Model file for the job. Use its own axes, mm. Face numbers are marked on the shaded views. A direction names the side the tool comes from. Coordinates: 2 decimals unless noted, no trailing zeros. Write each loop counter-clockwise with the first axis right and the second up, starting at its lowest first coordinate (ties: lowest second). Pieces come first, ordered by that corner, then holes.
Q1. Pin check, flat tips, straight feed: P1, Ø4, axis at x = 37, z = -152.5, coming from the -Y side; P2, Ø1, axis at x = -15.5, y = 946, coming from the +Z side. Stop position of each tip, or through.
Q2. Band-saw the part on C-C, the plane x = 33. Write the cut outline in (y, z), plus the area to 3 significant figures.
Q3. Band-saw the part on B-B, the plane y = 1525. Write the cut outline in (x, z), plus the area to 3 significant figures.
Q4. Pull direction X, two halves, no side cores. Call the marked faces 1, 2 and 3: released by +X, released by -X, zero draft, split by the parting line, or undercut.
Q5. Drill centre lines: probe 1 along Y at (x, z) = (62, -112); probe 2 along X at (y, z) = (1181, -19.5); probe 3 along Z at (x, y) = (-39.5, 1463). Where is each one in solid material? Low to high.
Q6. Band-saw the part on A-A, the plane z = -28.5. Write the cut outline in (x, y).
Q7. Which spindle directions (+Z, -Z, +X, -X, +Y, -Y) get a long thin tool onto all of the face, cutting with end or side? Do the marked faces 4 and 5. Say none if no direction does.
Autodesk Inventor part; units mm, degrees
ref_plane "YZ Plane" through (0, 0, 0) normal (1, 0, 0) x (0, 1, 0)
ref_plane "XZ Plane" through (0, 0, 0) normal (0, 1, 0) x (-1, 0, 0)
ref_plane "XY Plane" through (0, 0, 0) normal (0, 0, 1) x (1, 0, 0)
sketch "Schizzo1" plane through (0, 0, 0) normal (0, 0, 1) x (1, 0, 0)
  line L0 (-87.5, 0) -> (87.5, 0)
  line L1 (87.5, 0) -> (87.5, 2100)
  line L2 (87.5, 2100) -> (-87.5, 2100)
  line L3 (-87.5, 2100) -> (-87.5, 0)
  point P0 (0, 0)
  point P1 (0, 0)
  dimension "d0" = 175
  dimension "d1" = 2100
extrude "Estrusione1" add sketch "Schizzo1" against normal blind 200
shell "Svuotamento1" thickness 18 removed faces 1 at (-29.1667, 1400, 0)
sketch "Schizzo2" plane through (0, 0, 0) normal (0, 0, 1) x (1, 0, 0)
  line L0 (-69.5, 18) -> (-69.5, 2082)
  line L1 (69.5, 2082) -> (69.5, 18)
  line L2 (-69.5, 1632) -> (69.5, 1632)
  line L3 (69.5, 1632) -> (69.5, 1614)
  line L4 (69.5, 1614) -> (-69.5, 1614)
  line L5 (-69.5, 1614) -> (-69.5, 1632)
  line L6 (-69.5, 1164) -> (69.5, 1164)
  line L7 (69.5, 1164) -> (69.5, 1146)
  line L8 (69.5, 1146) -> (-69.5, 1146)
  line L9 (-69.5, 1146) -> (-69.5, 1164)
  line L10 (-69.5, 18) -> (-69.5, 2082)
  line L11 (69.5, 2082) -> (69.5, 18)
  line L12 (-69.5, 696) -> (69.5, 696)
  line L13 (69.5, 696) -> (69.5, 18)
  line L14 (69.5, 18) -> (-69.5, 18)
  line L15 (-69.5, 18) -> (-69.5, 696)
  point P0 (0, 0)
  point P1 (69.5, 1614)
  point P2 (69.5, 1632)
  point P3 (-69.5, 1632)
  point P4 (69.5, 1146)
  point P5 (69.5, 1164)
  point P6 (-69.5, 1164)
  point P7 (69.5, 18)
  dimension "d6" = 18
  dimension "d7" = 450
  dimension "d8" = 450
  dimension "d12" = 450
  dimension "d13" = 678
extrude "Estrusione2" add sketch "Schizzo2" against normal up to surface (182 mm away) contours L0 L12 L1 L14 | L0 L6 L1 L8 | L0 L2 L1 L4
equation "\"d8\" = d7"
equation "\"d12\" = d7"
properties part number "Mobiletto verticale"
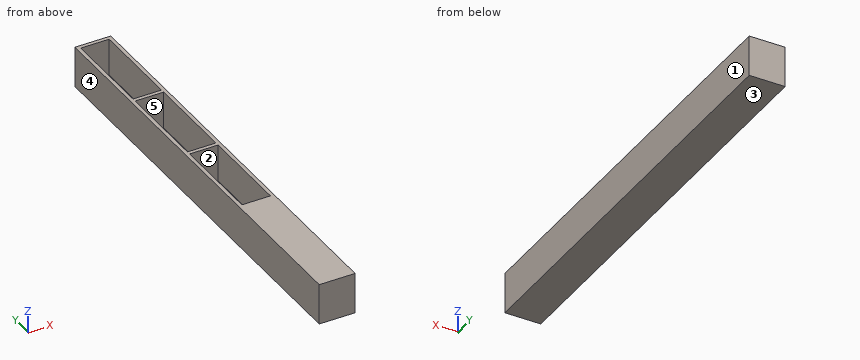
Answer sheet:
1. P1: stops at y = 0
1. P2: stops at z = -182
2. outline: (0, -200) - (2100, -200) - (2100, 0) - (2082, 0) - (2082, -182) - (1632, -182) - (1632, 0) - (1614, 0) - (1614, -182) - (1164, -182) - (1164, 0) - (1146, 0) - (1146, -182) - (696, -182) - (696, 0) - (0, 0) - close
2. area: 174,000 mm2
3. outline: (-87.5, -200) - (87.5, -200) - (87.5, 0) - (69.5, 0) - (69.5, -182) - (-69.5, -182) - (-69.5, 0) - (-87.5, 0) - close
3. area: 9,700 mm2
4. face 1: released by +X
4. face 2: undercut
4. face 3: zero draft
5. probe 1: y = 0 to 696, 1146 to 1164, 1614 to 1632, 2082 to 2100
5. probe 2: x = -87.5 to -69.5, 69.5 to 87.5
5. probe 3: z = -200 to -182
6. outline: (-87.5, 0) - (87.5, 0) - (87.5, 2100) - (-87.5, 2100) - close; hole (-69.5, 696) - (69.5, 696) - (69.5, 1146) - (-69.5, 1146) - close; hole (-69.5, 1164) - (69.5, 1164) - (69.5, 1614) - (-69.5, 1614) - close; hole (-69.5, 1632) - (69.5, 1632) - (69.5, 2082) - (-69.5, 2082) - close
7. face 4: +Z, -Z, -X, +Y, -Y
7. face 5: +Z
